Geometry check sheet. Reference: the model listing, model coordinates, mm. Give positions to 0.01 mm unless a question says otherwise; leave off trailing zeros. Use a Markdown table: item, result. Add a question column.
1. Cross-section at A-A on y = 1.6. Count the separate pieces of the cut face and the enclosed holes in it, and give its area (3 significant figures).
2. Draft check along X on faces 1 (the cylindrical face through (-1.33, 2.22, -34.51)), 2 (the flat face through (65, 2, 1)), 3 (the flat face through (-65, 2, 1)), 4 (the flat face through (-1, 4.5, -1)). Enter one of: pulls with the +X half, pulls with the -X half, needs draft (parallel to the pull), parting line crosses it, or undercut.
3. Material ranges on L1, parallel to X at y = 1.8, z = -39.68; L2, parallel to Z at x = -37.8, y = 1.6; L3, parallel to X at y = 0.95, z = 95, recorded low to high.
4. Depth check by flat-ended pin: P1, Ø4, axis at x = 60, z = 95, coming from the +Y side. Enter the tip coordinate at first touch or a pass-through.
from build123d import *

# Parameters (mm, degrees)
SKETCH1_W           = 130
SKETCH1_H           = 200
BOSS_EXTRUDE1_DEPTH = 4.5
SKETCH3_R           = 1.6
CUT_EXTRUDE1_DEPTH  = 4.5
SKETCH4_R           = 1.6
CUT_EXTRUDE2_DEPTH  = 4.5
SKETCH5_R           = 1.6
CUT_EXTRUDE3_DEPTH  = 4.5
SKETCH6_R           = 1.6
CUT_EXTRUDE4_DEPTH  = 4.5
SKETCH7_R           = 1.6
CUT_EXTRUDE5_DEPTH  = 4.5
SKETCH9_R           = 1.6
SKETCH9_R_2         = 10.25
CUT_EXTRUDE6_DEPTH  = 4.5


with BuildPart() as part:
    # Sketch1 → Boss-Extrude1 (new body)
    with BuildSketch(Plane(origin=(0, 0, 0), x_dir=(1, 0, 0), z_dir=(0, 1, 0))):
        Rectangle(SKETCH1_W, SKETCH1_H)
    extrude(amount=BOSS_EXTRUDE1_DEPTH)

    # Sketch3 → Cut-Extrude1 (cut)
    with BuildSketch(Plane(origin=(0, 0, 0), x_dir=(1, 0, 0), z_dir=(0, 1, 0))):
        with Locations((-60, -95)):
            Circle(SKETCH3_R)
        with Locations((60, -95)):
            Circle(SKETCH3_R)
        with Locations((-60, -60)):
            Circle(SKETCH3_R)
        with Locations((60, -60)):
            Circle(SKETCH3_R)
    extrude(amount=CUT_EXTRUDE1_DEPTH, mode=Mode.SUBTRACT)

    # Sketch4 → Cut-Extrude2 (cut)
    with BuildSketch(Plane(origin=(0, 0, 0), x_dir=(1, 0, 0), z_dir=(0, 1, 0))):
        with Locations((-35.055, 15.432)):
            Circle(SKETCH4_R)
        with Locations((36.957, 7.29)):
            Circle(SKETCH4_R)
        with Locations((36.445, 91.87)):
            Circle(SKETCH4_R)
        with Locations((-35.945, 92.13)):
            Circle(SKETCH4_R)
    extrude(amount=CUT_EXTRUDE2_DEPTH, mode=Mode.SUBTRACT)

    # Sketch5 → Cut-Extrude3 (cut)
    with BuildSketch(Plane(origin=(0, 0, 0), x_dir=(1, 0, 0), z_dir=(0, 1, 0))):
        with Locations((37.8, -12.298)):
            Circle(SKETCH5_R)
        with Locations((37.8, -42.298)):
            Circle(SKETCH5_R)
        with Locations((-37.8, -42.298)):
            Circle(SKETCH5_R)
        with Locations((-37.8, -12.298)):
            Circle(SKETCH5_R)
    extrude(amount=CUT_EXTRUDE3_DEPTH, mode=Mode.SUBTRACT)

    # Sketch6 → Cut-Extrude4 (cut)
    with BuildSketch(Plane(origin=(0, 0, 0), x_dir=(1, 0, 0), z_dir=(0, 1, 0))):
        with Locations((54.21, 79.68)):
            Circle(SKETCH6_R)
        with Locations((26.904, 96.063)):
            Circle(SKETCH6_R)
        with Locations((26.904, 56.063)):
            Circle(SKETCH6_R)
        with Locations((54.21, 39.68)):
            Circle(SKETCH6_R)
        with Locations((-54.21, 96.063)):
            Circle(SKETCH6_R)
        with Locations((-26.904, 79.68)):
            Circle(SKETCH6_R)
        with Locations((-54.21, 56.063)):
            Circle(SKETCH6_R)
        with Locations((-26.904, 39.68)):
            Circle(SKETCH6_R)
    extrude(amount=CUT_EXTRUDE4_DEPTH, mode=Mode.SUBTRACT)

    # Sketch7 → Cut-Extrude5 (cut)
    with BuildSketch(Plane(origin=(0, 0, 0), x_dir=(1, 0, 0), z_dir=(0, 1, 0))):
        with Locations((-8.1915, 69.312)):
            Circle(SKETCH7_R)
        with Locations((8.1915, 96.618)):
            Circle(SKETCH7_R)
        with Locations((16.8085, 69.312)):
            Circle(SKETCH7_R)
        with Locations((33.1915, 96.618)):
            Circle(SKETCH7_R)
        with Locations((41.8085, 69.312)):
            Circle(SKETCH7_R)
        with Locations((58.1915, 96.618)):
            Circle(SKETCH7_R)
        with Locations((-33.1915, 69.312)):
            Circle(SKETCH7_R)
        with Locations((-16.8085, 96.618)):
            Circle(SKETCH7_R)
        with Locations((-58.1915, 69.312)):
            Circle(SKETCH7_R)
        with Locations((-41.8085, 96.618)):
            Circle(SKETCH7_R)
    extrude(amount=CUT_EXTRUDE5_DEPTH, mode=Mode.SUBTRACT)

    # Sketch9 → Cut-Extrude6 (cut)
    with BuildSketch(Plane(origin=(0, 0, 0), x_dir=(1, 0, 0), z_dir=(0, 1, 0))):
        with Locations((0, -70)):
            Circle(SKETCH9_R)
        with Locations((0, -85)):
            Circle(SKETCH9_R)
        with Locations((0, 24.345540537)):
            Circle(SKETCH9_R_2)
        with Locations((17.5, 24.345540537)):
            Circle(SKETCH9_R)
        with Locations((-17.5, 24.345540537)):
            Circle(SKETCH9_R)
    extrude(amount=CUT_EXTRUDE6_DEPTH, mode=Mode.SUBTRACT)


solid = part.part
Values found:
| question | item | result |
|---|---|---|
| 1 | separate pieces | 1 |
| 1 | enclosed holes | 35 |
| 1 | area | 25,400 mm2 |
| 2 | face 1 | undercut |
| 2 | face 2 | pulls with the +X half |
| 2 | face 3 | pulls with the -X half |
| 2 | face 4 | needs draft |
| 3 | L1 | x = -65 to -28.5, -25.3 to 52.61, 55.81 to 65 |
| 3 | L2 | z = -100 to 10.7, 13.9 to 40.7, 43.9 to 100 |
| 3 | L3 | x = -65 to -61.6, -58.4 to 58.4, 61.6 to 65 |
| 4 | P1 | stops at y = 4.5 |
